Can you work these out from the model? Positions are in its coordinate system, mm. A direction names the side the tool comes from. Round coordinates to 2 decimals unless told otherwise and drop trailing zeros. Loops run counter-clockwise (first coordinate to the right, second up) from the corner with the lowest first, then second, coordinate; pieces in that order, holes last. Notation, with made-up numbers: (37, 70.5) - (52, 70.5) arc R15 ccw to (52, 76.5) - close; hole circle Ø6 at (30.5, 19.5). An arc over 180 degrees is marked (long way). Answer as CSV lines item,"result".
```python
from build123d import *

# Parameters (mm, degrees)
BOSS_EXTRUDE1_DEPTH = 11.09
SKETCH3_R           = 1.5
CUT_EXTRUDE4_DEPTH  = 10
SKETCH4_R           = 2.75
CUT_EXTRUDE3_DEPTH  = 2.5


with BuildPart() as part:
    # Sketch1 → Boss-Extrude1 (new body)
    with BuildSketch(Plane.XY):
        with BuildLine():
            Line((-8.04, 0), (-13.15, 0))
            Line((-13.15, 0), (-11.749422053, 4.05659727))
            ThreePointArc((-11.749422053, 4.05659727), (2.056645798, 12.258674809), (12.43, 0))
            Line((12.43, 0), (8.04, 0))
            ThreePointArc((8.04, 0), (5.685138521, 5.685138521), (0, 8.04))
            ThreePointArc((0, 8.04), (-5.685138521, 5.685138521), (-8.04, 0))
        make_face()
    extrude(amount=BOSS_EXTRUDE1_DEPTH)

    # Sketch3 → Cut-Extrude4 (cut)
    with BuildSketch(Plane.XZ):
        with Locations((-10.595, 5.95)):
            Circle(SKETCH3_R)
        with Locations((10.235, 5.545)):
            Circle(SKETCH3_R)
    extrude(amount=-CUT_EXTRUDE4_DEPTH, mode=Mode.SUBTRACT)

    # Sketch4 → Cut-Extrude3 (cut, symmetric)
    with BuildSketch(Plane(origin=(0, 9.5, 0), x_dir=(1, 0, 0), z_dir=(0, 1, 0))):
        with Locations((-10.595, -5.95)):
            Circle(SKETCH4_R)
        with Locations((10.235, -5.545)):
            Circle(SKETCH4_R)
    extrude(amount=CUT_EXTRUDE3_DEPTH, both=True, mode=Mode.SUBTRACT)


solid = part.part
```
Q1. Imagine slicing it at A-A (y = 3.25). Write out the boundary of the cut face in (x, z) (3 decimals), then the cut area to 3 significant figures.
Checks:
outline,"(-12.028, 0) - (-7.354, 0) - (-7.354, 11.09) - (-12.028, 11.09) - (-12.028, 6.394) arc R1.5 cw (long way) to (-12.028, 5.506) - close; (7.354, 0) - (11.998, 0) - (11.998, 11.09) - (7.354, 11.09) - close; hole circle Ø3 at (10.235, 5.545)"
area,"89.2 mm²"
Q2. If I drill on line 1 along X through (y, z) = (2, 6); line 2 along Y through (x, z) = (-9, 7.5); line 3 along X through (y, z) = (3.25, 5.95) (3 decimals), over which ranges is the centre line in solid material (lowest first)? Write a range as [from, to].
Checks:
line 1,"[-12.46, -12.09], [-9.1, -7.79], [7.79, 8.81], [11.66, 12.27]"
line 2,"[0, 7]"
line 3,"[-9.095, -7.354], [7.354, 8.791], [11.679, 11.998]"
Q3. On a 3-axis mill with a long thin cutter (end or side, diameter ignored), from which of +Z, -Z, +X, -X, +Y, -Y can I reach the whole of each face in a straight line? I mean faces 1 (the flat face through (8.5, 7, 5.5)), 2 (the cylindrical face through (-9.2, 2.7, 5.4)), 3 (the flat face through (-8.8, 7, 5.9)). Say none if no direction works.
Checks:
face 1,"+X, +Y"
face 2,"+Y, -Y"
face 3,"-X, +Y"
Q4. We'd pull the mould along Z, two halves only. Please class faces 4 (the cylindrical face through (8.736, 3.451, 5.611)), 5 (the flat face through (11, 0, 4)), 6 (the flat face through (0, 9, 0)): pulls with the +Z half, pulls with the -Z half, needs draft (parallel to the pull), parting line crosses it, or undercut.
Checks:
face 4,"undercut"
face 5,"needs draft"
face 6,"pulls with the -Z half"
Q5. I'm going to push flat-ended pins straight in: pin 1 Ø5 at (x, z) = (-4.5, 3) entering from +Y; pin 2 Ø0.7 at (x, z) = (-9, 6.5) entering from +Y; pin 3 Ø2.5 at (x, z) = (10.235, 5.545) entering from -Y; pin 4 Ø6 at (y, z) = (7.5, 4.5) entering from -X. Where does each tip first touch, or does it pass through?
Checks:
pin 1,"y = 12.27"
pin 2,"y = 7"
pin 3,"through"
pin 4,"x = -11.59"
Q6. Imagine slicing it at B-B (y = 6.5). Write out the boundary of the cut face in (x, z) (3 decimals), then the cut area to 3 significant figures.
Checks:
outline,"(-10.595, 0) - (-4.732, 0) - (-4.732, 11.09) - (-10.595, 11.09) - (-10.595, 7.45) arc R1.5 cw to (-10.595, 4.45) - close; (4.732, 0) - (10.595, 0) - (10.595, 4.089) arc R1.5 cw (long way) to (10.595, 7.001) - (10.595, 11.09) - (4.732, 11.09) - close"
area,"122 mm²"
Q7. Imagine slicing it at D-D (x = -10). Write out the boundary of the cut face in (y, z).
Checks:
outline,"(0, 0) - (7.38, 0) - (7.38, 3.27) - (7, 3.27) - (7, 4.57) - (0, 4.57) - close; (0, 7.33) - (7, 7.33) - (7, 8.63) - (7.38, 8.63) - (7.38, 11.09) - (0, 11.09) - close"
Q8. Imagine slicing it at C-C (z = 5.95). Write out the boundary of the cut face in (x, y) (3 decimals).
Checks:
outline,"(-13.15, 0) - (-12.095, 0) - (-12.095, 3.056) - close; (-9.095, 0) - (-8.04, 0) arc R8.04 cw to (8.04, 0) - (8.791, 0) - (8.791, 7) - (7.515, 7) - (7.515, 9.901) arc R12.43 ccw to (-7.845, 9.642) - (-7.845, 7) - (-9.095, 7) - close; (11.679, 0) - (12.43, 0) arc R12.43 ccw to (11.679, 4.254) - close"
